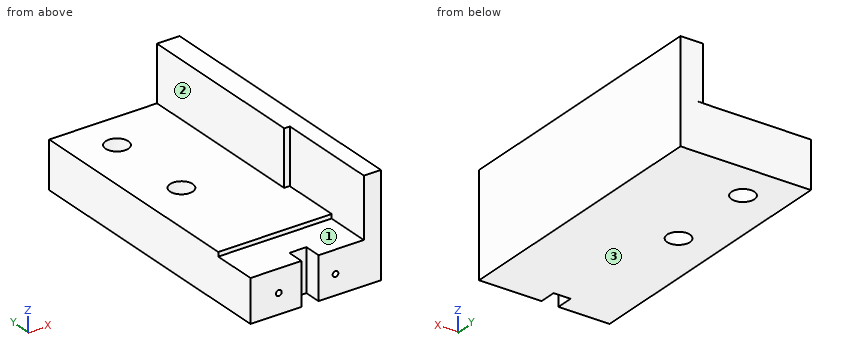
```python
from build123d import *

# Parameters (mm, degrees)
BOSS_EXTRUDE1_DEPTH = 50
SKETCH4_W           = 20
SKETCH4_H           = 1.5
CUT_EXTRUDE1_DEPTH  = 8
SKETCH5_R           = 0.5
CUT_EXTRUDE2_DEPTH  = 8
SKETCH6_W           = 3
SKETCH6_H           = 3
CUT_EXTRUDE3_DEPTH  = 7.5
SKETCH7_R           = 2
CUT_EXTRUDE4_DEPTH  = 9
SKETCH8_W           = 20
SKETCH8_H           = 42
CUT_EXTRUDE5_DEPTH  = 0.75
SKETCH9_W           = 9.72
SKETCH9_H           = 31.616710758
BOSS_EXTRUDE2_DEPTH = 1


with BuildPart() as part:
    # Sketch3 → Boss-Extrude1 (new body)
    with BuildSketch(Plane(origin=(0, 0, 0), x_dir=(1, 0, 0), z_dir=(0, 1, 0))):
        Polygon((0, 0), (0, 9), (23, 9), (23, -9), (20, -9), (20, 0), align=None)
    extrude(amount=BOSS_EXTRUDE1_DEPTH)

    # Sketch4 → Cut-Extrude1 (cut)
    with BuildSketch(Plane.XZ):
        with Locations((10, -0.75)):
            Rectangle(SKETCH4_W, SKETCH4_H)
    extrude(amount=-CUT_EXTRUDE1_DEPTH, mode=Mode.SUBTRACT)

    # Sketch5 → Cut-Extrude2 (cut)
    with BuildSketch(Plane.XZ):
        with Locations(Location((5, -5.5, 0), (0, 0, 270))):
            Circle(SKETCH5_R)
        with Locations(Location((15, -5.5, 0), (0, 0, 270))):
            Circle(SKETCH5_R)
    extrude(amount=-CUT_EXTRUDE2_DEPTH, mode=Mode.SUBTRACT)

    # Sketch6 → Cut-Extrude3 (cut)
    with BuildSketch(Plane.XY.offset(-1.5)):
        with Locations((10.5, 1.5)):
            Rectangle(SKETCH6_W, SKETCH6_H)
    extrude(amount=-CUT_EXTRUDE3_DEPTH, mode=Mode.SUBTRACT)

    # Sketch7 → Cut-Extrude4 (cut)
    with BuildSketch(Plane(origin=(0, 0, -9), x_dir=(-1, 0, 0), z_dir=(0, 0, -1))):
        with Locations((-7, 27)):
            Circle(SKETCH7_R)
        with Locations((-7, 43)):
            Circle(SKETCH7_R)
    extrude(amount=-CUT_EXTRUDE4_DEPTH, mode=Mode.SUBTRACT)

    # Sketch8 → Cut-Extrude5 (cut)
    with BuildSketch(Plane.XY):
        with Locations((10, 29)):
            Rectangle(SKETCH8_W, SKETCH8_H)
    extrude(amount=-CUT_EXTRUDE5_DEPTH, mode=Mode.SUBTRACT)

    # Sketch9 → Boss-Extrude2 (add)
    with BuildSketch(Plane.ZY.offset(-20)):
        with Locations((4.14, 34.191644621)):
            Rectangle(SKETCH9_W, SKETCH9_H)
    extrude(amount=BOSS_EXTRUDE2_DEPTH)


solid = part.part
```
Check sheet for the modelled part. Datum: model origin and axes. Units: mm. Face numbers are marked on the shaded views. A direction names the side the tool comes from. Coordinates: 2 decimals unless noted, no trailing zeros. Write each loop counter-clockwise with the first axis right and the second up, starting at its lowest first coordinate (ties: lowest second). Pieces come first, ordered by that corner, then holes. Notation, with made-up numbers: (-5, 52) - (17, 52) arc R16 cw to (17, 61) - close; hole circle Ø2 at (35, 26). An arc over 180 degrees is marked (long way). One line per question, with ' | ' between items.
Item 1: Thickness scan on line 1 (X direction, y = 5, z = -5.5); line 2 (Y direction, x = 7, z = -6); line 3 (X direction, y = 20, z = 2). Record the ranges inside material, lowest first. Write a range as [from, to].
Determined:
line 1: x = [0, 4.5], [5.5, 14.5], [15.5, 23] | line 2: y = [0, 25], [29, 41], [45, 50] | line 3: x = [19, 23]
Item 2: Gauge pin test, flat ends, axial feed: P1, Ø0.9, axis at x = 11, z = -6.5, coming from the -Y side; P2, Ø5, axis at y = 13, z = 5.5, coming from the -X side; P3, Ø5, axis at x = 13.5, y = 41, coming from the +Z side; P4, Ø2.5, axis at x = 7, y = 43, coming from the -Z side. Record the tip position at first contact, or that the pin passes through.
Determined:
P1: stops at y = 3 | P2: stops at x = 20 | P3: stops at z = -0.75 | P4: passes through
Item 3: Sectioned sample at C-C on x = 8. Record the boundary of the cut face in (y, z), plus the area to 3 significant figures.
Determined:
outline: (0, -9) - (25.27, -9) - (25.27, -0.75) - (8, -0.75) - (8, -1.5) - (0, -1.5) - close; (28.73, -9) - (41.27, -9) - (41.27, -0.75) - (28.73, -0.75) - close; (44.73, -9) - (50, -9) - (50, -0.75) - (44.73, -0.75) - close | area: 349 mm2
Item 4: Sectioned sample at D-D on z = 6. Record the boundary of the cut face in (x, y), plus the area to 3 significant figures.
Determined:
outline: (19, 18.38) - (20, 18.38) - (20, 0) - (23, 0) - (23, 50) - (19, 50) - close | area: 182 mm2
Item 5: Access from +Z, -Z, +X, -X, +Y, -Y to the whole of each face (thin tool, end or side, straight path). Record for the marked faces 1, 2 and 3.
Determined:
face 1: +Z, -X, -Y | face 2: +Z, -X, +Y, -Y | face 3: -Z, +X, -X, +Y, -Y
Item 6: Sectioned sample at B-B on x = 15. Record the boundary of the cut face in (y, z), plus the area to 4 significant figures.
Determined:
outline: (0, -9) - (50, -9) - (50, -0.75) - (8, -0.75) - (8, -1.5) - (0, -1.5) - (0, -5) - (8, -5) - (8, -6) - (0, -6) - close | area: 398.5 mm2
